Here's how the part is built. I have some questions about the finished solid (model axes, mm). Face numbers are marked on the shaded views. A direction names the side the tool comes from. Give positions to 0.01 mm unless a question says otherwise; leave off trailing zeros. Write each loop counter-clockwise with the first axis right and the second up, starting at its lowest first coordinate (ties: lowest second). Pieces come first, ordered by that corner, then holes. Notation, with made-up numbers: (-31, -3) -> (-17, -3) arc R13 cw to (-17, 15) -> close; hole circle Ø3 at (42.5, 18). An arc over 180 degrees is marked (long way). Use CSV: the item, a comma, the result in double quotes. Start each with the question number.
(1) For pin 1 Ø3 at (x, z) = (3, -3) entering from +Y, with a flat end and sliding along its axis, tell me the tip position at first contact or that it passes through.
(2) Which directions (+Z, -Z, +X, -X, +Y, -Y) give clear straight access to the entire face, cutting with the end or side of a thin tool? Please do the marked faces 1 and 2.
(3) Suppose I cut it at D-D on z = 0.75. List the corners of the cut face in (x, y) for me, plus the area to 3 significant figures.
(4) I need wall thicknesses on L1, parallel to Z at x = 1, y = -2; L2, parallel to Y at x = 1.75, z = -0.5. Which ranges of each line are inside material? Lowest first, please. Write a range as [from, to].
(5) Suppose I cut it at C-C on z = -2.5. List the corners of the cut face in (x, y) for me, plus the area to 3 significant figures.
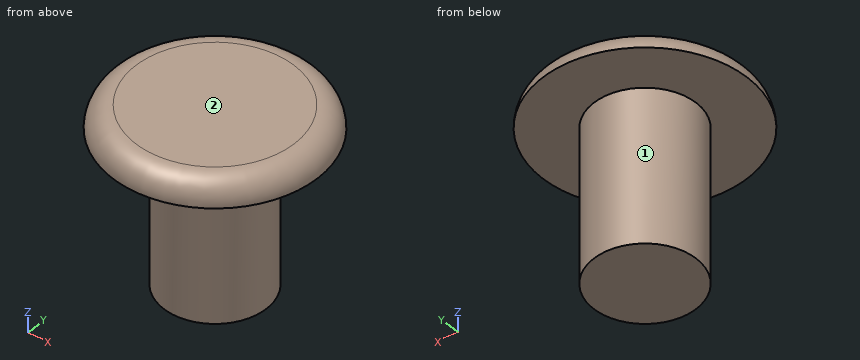
Autodesk Inventor part; units mm, degrees
ref_plane "YZ Plane" through (0, 0, 0) normal (1, 0, 0) x (0, 1, 0)
ref_plane "XZ Plane" through (0, 0, 0) normal (0, 1, 0) x (-1, 0, 0)
ref_plane "XY Plane" through (0, 0, 0) normal (0, 0, 1) x (1, 0, 0)
sketch "スケッチ1" plane through (0, 0, 0) normal (0, 0, 1) x (1, 0, 0)
  circle A0 centre (0, 0) radius 4
  dimension "d0" = 8
extrude "押し出し1" add sketch "スケッチ1" along normal blind 0.9
sketch "スケッチ2" plane through (0, 0, 0) normal (0, 0, -1) x (-1, 0, 0)
  circle A0 centre (0, 0) radius 2
  dimension "d3" = 4
extrude "押し出し2" add sketch "スケッチ2" along normal blind 6
thread "ねじ1"
fillet "フィレット1" radius 0.9 1 edges at (-4, 0, 0.9)
properties part number "ネジ低頭m4.06" material "鋼 AISI 4340 242 HR"
Geometry says:
1,pin 1,"y = 1.32"
2,face 1,"-Z"
2,face 2,"+Z, +X, -X, +Y, -Y"
3,outline,"circle Ø7.2 at (0, 0)"
3,area,"40.7 mm²"
4,L1,"[0, 0.9]"
4,L2,"[-0.97, 0.97]"
5,outline,"circle Ø4 at (0, 0)"
5,area,"12.6 mm²"
